Check sheet for the modelled part. Datum: model origin and axes. Units: mm. A direction names the side the tool comes from. Coordinates: 2 decimals unless noted, no trailing zeros. Loops run counter-clockwise (first coordinate to the right, second up) from the corner with the lowest first, then second, coordinate; pieces in that order, holes last.
```python
from build123d import *

# Parameters (mm, degrees)
SKETCH_2_R          = 1.6
SKETCH_2_R_2        = 17
SKETCH_2_R_3        = 1.65
EXTRUDE_2_DEPTH     = 13
CUT_EXTRUDE_1_DEPTH = 3
EXTRUDE_3_DEPTH     = 20
CUT_EXTRUDE_2_DEPTH = 125.506947597
SKETCH_8_W          = 24
SKETCH_8_H          = 20
CUT_EXTRUDE_3_DEPTH = 6
SKETCH_10_R         = 3
SKETCH_10_R_2       = 1.65
CUT_EXTRUDE_4_DEPTH = 5


with BuildPart() as part:
    # 草图2 → 凸台-拉伸2 (new body)
    with BuildSketch(Plane(origin=(0, 0, 0), x_dir=(1, 0, 0), z_dir=(0, 1, 0))):
        Polygon((-44.3, 33.8), (-44.3, 74.3), (-29.3, 74.3), (-29.3, 53.8), (12.5, 53.8), (12.5, 61.8), (37.5, 61.8), (37.5, 53.8), (79.3, 53.8), (79.3, 74.3), (94.3, 74.3), (94.3, 33.8), (50, 33.8), (50, 0), (0, 0), (0, 33.8), align=None)
        with Locations(Location((-36.8, 69.8, 0), (0, 0, 90))):
            Circle(SKETCH_2_R, mode=Mode.SUBTRACT)
        with Locations(Location((-36.8, 56.2, 0), (0, 0, 90))):
            Circle(SKETCH_2_R, mode=Mode.SUBTRACT)
        with Locations(Location((86.8, 69.8, 0), (0, 0, 90))):
            Circle(SKETCH_2_R, mode=Mode.SUBTRACT)
        with Locations(Location((86.8, 56.2, 0), (0, 0, 90))):
            Circle(SKETCH_2_R, mode=Mode.SUBTRACT)
        with Locations(Location((18, 56.2, 0), (0, 0, 90))):
            Circle(SKETCH_2_R, mode=Mode.SUBTRACT)
        with Locations(Location((32, 56.2, 0), (0, 0, 90))):
            Circle(SKETCH_2_R, mode=Mode.SUBTRACT)
        with Locations(Location((25, 28.8, 0), (0, 0, 90))):
            Circle(SKETCH_2_R_2, mode=Mode.SUBTRACT)
        with Locations(Location((40.5, 44.3, 0), (0, 0, 90))):
            Circle(SKETCH_2_R_3, mode=Mode.SUBTRACT)
        with Locations(Location((40.5, 13.3, 0), (0, 0, 90))):
            Circle(SKETCH_2_R_3, mode=Mode.SUBTRACT)
        with Locations(Location((9.5, 13.3, 0), (0, 0, 90))):
            Circle(SKETCH_2_R_3, mode=Mode.SUBTRACT)
        with Locations(Location((9.5, 44.3, 0), (0, 0, 90))):
            Circle(SKETCH_2_R_3, mode=Mode.SUBTRACT)
    extrude(amount=EXTRUDE_2_DEPTH)

    # 草图3 → 切除-拉伸1 (cut)
    with BuildSketch(Plane(origin=(0, 13, 0), x_dir=(1, 0, 0), z_dir=(0, 1, 0))):
        Polygon((21.464101615, 56.2), (19.732050808, 59.2), (16.267949192, 59.2), (14.535898385, 56.2), (16.267949192, 53.2), (19.732050808, 53.2), align=None)
        Polygon((35.464101615, 56.2), (33.732050808, 59.2), (30.267949192, 59.2), (28.535898385, 56.2), (30.267949192, 53.2), (33.732050808, 53.2), align=None)
    extrude(amount=-CUT_EXTRUDE_1_DEPTH, mode=Mode.SUBTRACT)

    # 草图6 → 凸台-拉伸3 (add)
    with BuildSketch(Plane(origin=(0, 13, 0), x_dir=(1, 0, 0), z_dir=(0, 1, 0))):
        Polygon((0, 33.8), (0, 0), (50, 0), (50, 33.8), (47, 33.8), (47, 4), (3, 4), (3, 33.8), align=None)
    extrude(amount=EXTRUDE_3_DEPTH)

    # 草图7 → 切除-拉伸2 (cut, through all)
    with BuildSketch(Plane.ZY):
        Polygon((-33.8, 13), (-4, 33), (-33.8, 33), align=None)
    extrude(amount=-CUT_EXTRUDE_2_DEPTH, mode=Mode.SUBTRACT)

    # 草图8 → 切除-拉伸3 (cut)
    with BuildSketch(Plane(origin=(0, 13, 0), x_dir=(1, 0, 0), z_dir=(0, 1, 0))):
        with Locations((25, 14)):
            Rectangle(SKETCH_8_W, SKETCH_8_H)
    extrude(amount=-CUT_EXTRUDE_3_DEPTH, mode=Mode.SUBTRACT)

    # 草图10 → 切除-拉伸4 (cut)
    with BuildSketch(Plane.XY):
        with Locations((25, 17)):
            Circle(SKETCH_10_R)
        with Locations((30.173451969, 23.102081179)):
            Circle(SKETCH_10_R_2)
        with Locations((30.173451969, 12.264714161)):
            Circle(SKETCH_10_R_2)
        with Locations((19.336084951, 12.264714161)):
            Circle(SKETCH_10_R_2)
        with Locations((19.336084951, 23.102081179)):
            Circle(SKETCH_10_R_2)
    extrude(amount=-CUT_EXTRUDE_4_DEPTH, mode=Mode.SUBTRACT)


solid = part.part
```
1) Mould release check, pull along Z, two halves, no side actions. Record for faces 1 (the flat face through (29.4, 11.5, -54.7)), 2 (the flat face through (-9, 6, -53.8)), 3 (the cylindrical face through (24.35, 14.07, -1.97)), 4 (the flat face through (15.4, 11.5, -54.7)): +Z half, -Z half, draft (parallel to the pull), parting line (faces both ways), or undercut.
Answer sheet:
face 1: undercut
face 2: -Z half
face 3: draft
face 4: undercut
2) Scan lines: line 1 (X direction, y = 6, z = -69.8); line 2 (X direction, y = 27.5, z = -6); line 3 (X direction, y = 4.75, z = -28.8). Record each from-to range of solid material in increasing order.
Answer sheet:
line 1: x = -44.3 to -38.4, -35.2 to -29.3, 79.3 to 85.2, 88.4 to 94.3
line 2: x = 0 to 3, 47 to 50
line 3: x = 0 to 8, 42 to 50
3) Section check A-A on x = 25. Enter the section's corners in (y, z), plus the area to 3 significant figures.
Answer sheet:
outline: (0, -61.8) - (13, -61.8) - (13, -45.8) - (0, -45.8) - close; (0, -11.8) - (7, -11.8) - (7, -4) - (14, -4) - (14, 0) - (0, 0) - close; (20, -4) - (33, -4) - (33, 0) - (20, 0) - close
area: 371 mm2
4) Depth check by flat-ended pin: pin 1 (1.8 mm diameter, centred on y = 10, z = -8.5, fed in from -X); pin 2 (6 mm diameter, centred on y = 19.5, z = -14.5, fed in from +X); pin 3 (5 mm diameter, centred on x = -36.8, z = -56.2, fed in from +Y). Enter the tip coordinate at first touch or a pass-through.
Answer sheet:
pin 1: stops at x = 0
pin 2: stops at x = 50
pin 3: stops at y = 13
5) Section check B-B on z = -69.8. Enter the section's corners in (x, y).
Answer sheet:
outline: (-44.3, 0) - (-38.4, 0) - (-38.4, 13) - (-44.3, 13) - close; (-35.2, 0) - (-29.3, 0) - (-29.3, 13) - (-35.2, 13) - close; (79.3, 0) - (85.2, 0) - (85.2, 13) - (79.3, 13) - close; (88.4, 0) - (94.3, 0) - (94.3, 13) - (88.4, 13) - close
6) Set-up check for faces 5 (the flat face through (32, 12, -53.2)), 6 (the flat face through (0, 13, -13)), 7 (the flat face through (50, 13, -13)): record each of +Z, -Z, +X, -X, +Y, -Y from which the full face is reachable in a straight line by a thin tool's end or side.
Answer sheet:
face 5: +Y
face 6: +Z, -X, +Y, -Y
face 7: +Z, +X, +Y, -Y
7) Section check C-C on y = 17. Enter the section's corners in (x, z).
Answer sheet:
outline: (0, -27.84) - (3, -27.84) - (3, -4) - (22, -4) - (22, 0) - (0, 0) - close; (28, -4) - (47, -4) - (47, -27.84) - (50, -27.84) - (50, 0) - (28, 0) - close
8) Section check D-D on z = -27. Enter the section's corners in (x, y).
Answer sheet:
outline: (0, 0) - (8.1, 0) - (8.1, 13) - (3, 13) - (3, 17.56) - (0, 17.56) - close; (41.9, 0) - (50, 0) - (50, 17.56) - (47, 17.56) - (47, 13) - (41.9, 13) - close
